Part model, mm, in its own coordinate system. A direction names the side the tool comes from. Give positions to 0.01 mm unless a question says otherwise; leave off trailing zeros. Write each loop counter-clockwise with the first axis right and the second up, starting at its lowest first coordinate (ties: lowest second). Pieces come first, ordered by that corner, then holes.
from build123d import *

# Parameters (mm, degrees)
SKETCH1_W           = 10
SKETCH1_H           = 25
BOSS_EXTRUDE1_DEPTH = 5
SKETCH2_W           = 10
SKETCH2_H           = 25
BOSS_EXTRUDE2_DEPTH = 1
SKETCH3_W           = 7
SKETCH3_H           = 5
CUT_EXTRUDE1_DEPTH  = 5


with BuildPart() as part:
    # Sketch1 → Boss-Extrude1 (new body)
    with BuildSketch(Plane.XY):
        with Locations((3.5, 11)):
            Rectangle(SKETCH1_W, SKETCH1_H)
        Polygon((7, 17), (3, 17), (3, 15), (7, 15), (7, 0), (0, 0), (0, 22), (7, 22), align=None, mode=Mode.SUBTRACT)
    extrude(amount=BOSS_EXTRUDE1_DEPTH)

    # Sketch2 → Boss-Extrude2 (add)
    with BuildSketch(Plane(origin=(0, 0, 0), x_dir=(-1, 0, 0), z_dir=(0, 0, -1))):
        with Locations((-3.5, 11)):
            Rectangle(SKETCH2_W, SKETCH2_H)
    extrude(amount=BOSS_EXTRUDE2_DEPTH)

    # Sketch3 → Cut-Extrude1 (cut)
    with BuildSketch(Plane(origin=(0, 0, 0), x_dir=(1, 0, 0), z_dir=(0, 1, 0))):
        with Locations((3.5, -2.5)):
            Rectangle(SKETCH3_W, SKETCH3_H)
    extrude(amount=-CUT_EXTRUDE1_DEPTH, mode=Mode.SUBTRACT)


solid = part.part
1) 3-axis set-ups, long thin cutter, end or side, ignore diameter. For faces 5 (the flat face through (5, 17, 2)), 6 (the flat face through (4, 11, -1)), 7 (the flat face through (3, 16, 2)): which of +Z, -Z, +X, -X, +Y, -Y reach the whole face in a straight line?
Check result:
face 5: +Z
face 6: -Z, +X, -X, +Y, -Y
face 7: +Z, -Y
2) Drill centre lines: L1, parallel to X at y = 18.25, z = 1.9; L2, parallel to Y at x = 3.5, z = 0.35; L3, parallel to Y at x = 0.75, z = 2.9. Where is each one in solid material? Low to high.
Check result:
L1: x = -1.5 to 0, 7 to 8.5
L2: y = 15 to 17, 22 to 23.5
L3: y = 22 to 23.5
3) Saw through at A-A (x = 4.5). Write the cut outline in (y, z).
Check result:
outline: (-1.5, -1) - (23.5, -1) - (23.5, 5) - (22, 5) - (22, 0) - (17, 0) - (17, 5) - (15, 5) - (15, 0) - (-1.5, 0) - close
4) Saw through at D-D (x = 1). Write the cut outline in (y, z), and give its area (3 significant figures).
Check result:
outline: (-1.5, -1) - (23.5, -1) - (23.5, 5) - (22, 5) - (22, 0) - (-1.5, 0) - close
area: 32.5 mm2
5) Saw through at C-C (z = 4.55). Write the cut outline in (x, y), and give its area (3 significant figures).
Check result:
outline: (-1.5, -1.5) - (0, -1.5) - (0, 22) - (7, 22) - (7, 17) - (3, 17) - (3, 15) - (7, 15) - (7, -1.5) - (8.5, -1.5) - (8.5, 23.5) - (-1.5, 23.5) - close
area: 93.5 mm2
6) Mould opens along X. For faces 1 (the flat face through (5, 15, 2)), 2 (the flat face through (4, 23.5, 2)), 3 (the flat face through (8.5, 11, 2)), 4 (the flat face through (-1.5, 11, 2)) say: +X half, -X half, draft (parallel to the pull), parting line (faces both ways), or undercut.
Check result:
face 1: undercut
face 2: draft
face 3: +X half
face 4: -X half
7) Saw through at B-B (y = 11.5). Write the cut outline in (x, z), and give its area (3 significant figures).
Check result:
outline: (-1.5, -1) - (8.5, -1) - (8.5, 5) - (7, 5) - (7, 0) - (0, 0) - (0, 5) - (-1.5, 5) - close
area: 25.0 mm2
